```python
from build123d import *

# Parameters (mm, degrees)
F2_DEPTH = 3.5
F3_DEPTH = 1


with BuildPart() as f2:
    # F1 (on face) → F2 (new body, symmetric)
    with BuildSketch(Plane.XZ):
        with BuildLine():
            Line((-2.286308, 32.102048), (-32.5, 5))
            Line((-32.5, 5), (-32.5, 0))
            Line((-32.5, 0), (32.5, 0))
            Line((32.5, 0), (32.5, 4))
            Line((32.5, 4), (17.657075, 28.696322))
            ThreePointArc((17.657075, 28.696322), (17.473375, 28.828507), (17.258243, 28.758243))
            Line((17.258243, 28.758243), (16.611408, 28.111408))
            ThreePointArc((16.611408, 28.111408), (16.489934, 28.044379), (16.351427, 28.052438))
            ThreePointArc((16.351427, 28.052438), (9.312089, 31.038714), (1.957773, 33.132551))
            ThreePointArc((1.957773, 33.132551), (-0.293903, 33.151198), (-2.286308, 32.102048))
        make_face()
        with BuildLine():
            Line((16.35495, 25.039163), (29.500001, 3.16784))
            Line((29.500001, 3.16784), (29.500001, 2.999999))
            Line((29.500001, 2.999999), (-29.500001, 2.999999))
            Line((-29.500001, 2.999999), (-29.500001, 3.66094))
            Line((-29.500001, 3.66094), (-0.283103, 29.868852))
            ThreePointArc((-0.283103, 29.868852), (0.435633, 30.241011), (1.244666, 30.217565))
            ThreePointArc((1.244666, 30.217565), (8.316297, 28.208802), (15.081898, 25.333087))
            ThreePointArc((15.081898, 25.333087), (15.703501, 25.121492), (16.35495, 25.039163))
        make_face(mode=Mode.SUBTRACT)
    extrude(amount=F2_DEPTH, both=True)

    # F1 (on face) → F3 (join, symmetric)
    with BuildSketch(Plane.XZ):
        with BuildLine():
            Line((29.500001, 2.999999), (29.500001, 3.16784))
            Line((29.500001, 3.16784), (16.35495, 25.039163))
            ThreePointArc((16.35495, 25.039163), (15.703501, 25.121492), (15.081898, 25.333087))
            ThreePointArc((15.081898, 25.333087), (8.316297, 28.208802), (1.244666, 30.217565))
            ThreePointArc((1.244666, 30.217565), (0.435633, 30.241011), (-0.283103, 29.868852))
            Line((-0.283103, 29.868852), (-29.500001, 3.66094))
            Line((-29.500001, 3.66094), (-29.500001, 2.999999))
            Line((-29.500001, 2.999999), (29.500001, 2.999999))
        make_face()
    extrude(amount=F3_DEPTH, both=True)


solid = f2.part
```
For this review, take the finished solid that the model builds, in its own axes (mm). A direction names the side the tool comes from. Round coordinates to 2 decimals unless told otherwise and drop trailing zeros. Loops run counter-clockwise (first coordinate to the right, second up) from the corner with the lowest first, then second, coordinate; pieces in that order, holes last.
Q1. Add section C-C on z = 8.5. Write out the cut boundary in (x, y).
Result sheet:
outline: (-28.6, -3.5) - (-24.11, -3.5) - (-24.11, -1) - (26.3, -1) - (26.3, -3.5) - (29.8, -3.5) - (29.8, 3.5) - (26.3, 3.5) - (26.3, 1) - (-24.11, 1) - (-24.11, 3.5) - (-28.6, 3.5) - close
Q2. Mouldability with a two-part tool opening along Z and no side actions: class faces 4 (the face through (-15.1, -2.27, 16.58)), 5 (the face through (-17.18, -0.05, 18.74)), 6 (the face through (0, -3.5, 2)), 7 (the face through (0, -1, 14)) as +Z half, -Z half, draft (parallel to the pull), parting line (faces both ways), or undercut.
Result sheet:
face 4: undercut
face 5: +Z half
face 6: draft
face 7: undercut
Q3. Insertion check: pin 1 Ø8 at (x, z) = (4, 18.5) entering from +Y; pin 2 Ø2 at (x, y) = (8.5, -2) entering from +Z; pin 3 Ø8 at (x, z) = (-2.5, 13) entering from -Y. Each pin has a flat end and moves straight along its axis. Give the tip position at first contact, or say it passes through.
Result sheet:
pin 1: stops at y = 1
pin 2: stops at z = 31.65
pin 3: stops at y = -1
Q4. To check wall thickness, follow line 1 along Y through (x, z) = (7, 17.5); line 2 along Z through (x, y) = (15, -0.5); line 3 along X through (y, z) = (-1.5, 21.5). State the ranges of each line that lie inside material, in increasing order.
Result sheet:
line 1: y = -1 to 1
line 2: z = 0 to 28.71
line 3: x = -14.11 to -9.61, 18.48 to 21.98
Q5. Add section A-A on y = -2. Write out the cut boundary in (x, z), plus the area to 3 significant figures.
Result sheet:
outline: (-32.5, 0) - (32.5, 0) - (32.5, 4) - (17.66, 28.7) arc R0.25 ccw to (17.26, 28.76) - (16.61, 28.11) arc R0.25 cw to (16.35, 28.05) arc R61.78 ccw to (1.96, 33.13) arc R4.61 ccw to (-2.29, 32.1) - (-32.5, 5) - close; hole (-29.5, 3) - (29.5, 3) - (29.5, 3.17) - (16.35, 25.04) arc R3.25 cw to (15.08, 25.33) arc R58.78 ccw to (1.24, 30.22) arc R1.61 ccw to (-0.28, 29.87) - (-29.5, 3.66) - close
area: 460 mm2
Q6. Machinability: for faces 1 (the face through (0, -2, 3)), 2 (the face through (8.219, 2.232, 28.243)), 3 (the face through (0, 3.5, 2)), which of the approach directions +Z, -Z, +X, -X, +Y, -Y give a long, thin tool a straight path to every point of the face, cutting with its end or side? Answer none if there is none.
Result sheet:
face 1: -Y
face 2: +Y
face 3: +Z, -Z, +X, -X, +Y
Q7. Add section B-B on x = -18.5. Write out the cut boundary in (y, z).
Result sheet:
outline: (-3.5, 0) - (3.5, 0) - (3.5, 3) - (1, 3) - (1, 13.53) - (3.5, 13.53) - (3.5, 17.56) - (-3.5, 17.56) - (-3.5, 13.53) - (-1, 13.53) - (-1, 3) - (-3.5, 3) - close
